from build123d import *

# Parameters (mm, degrees)
SKETCH1_R           = 48.26
SKETCH1_R_2         = 41.275
BOSS_EXTRUDE1_DEPTH = 12.7
SKETCH2_W           = 12.7
SKETCH2_H           = 12.7
BOSS_EXTRUDE2_DEPTH = 12.7
SKETCH4_W           = 2.54
SKETCH4_H           = 44.098902666
CUT_EXTRUDE2_DEPTH  = 79.456734484
BOSS_EXTRUDE3_REACH = 128.717
BOSS_EXTRUDE3_START = 48.26
SKETCH5_W           = 60.540412833
SKETCH5_H           = 12.7
SKETCH6_W           = 46.99
SKETCH6_H           = 50.8
BOSS_EXTRUDE4_DEPTH = 12.7
SKETCH7_R           = 3.429
SKETCH7_W           = 12.7
SKETCH7_H           = 11.43
CUT_EXTRUDE3_DEPTH  = 123.012315484


with BuildPart() as part:
    # Sketch1 → Boss-Extrude1 (new body)
    with BuildSketch(Plane(origin=(0, 0, 0), x_dir=(1, 0, 0), z_dir=(0, 1, 0))):
        with Locations(Location((0, 0, 0), (0, 0, 270))):
            Circle(SKETCH1_R)
        with Locations(Location((0, 0, 0), (0, 0, 270))):
            Circle(SKETCH1_R_2, mode=Mode.SUBTRACT)
    extrude(amount=BOSS_EXTRUDE1_DEPTH)

    # Sketch2 → Boss-Extrude2 (add)
    with BuildSketch(Plane(origin=(0, 0, 0), x_dir=(1, 0, 0), z_dir=(0, 1, 0))):
        with Locations((0, 54.190412833)):
            Rectangle(SKETCH2_W, SKETCH2_H)
    extrude(amount=BOSS_EXTRUDE2_DEPTH)

    # Sketch4 → Cut-Extrude2 (cut, through all)
    with BuildSketch(Plane(origin=(0, 0, 0), x_dir=(1, 0, 0), z_dir=(0, 1, 0))):
        with Locations((0, 60.121342859)):
            Rectangle(SKETCH4_W, SKETCH4_H)
    extrude(amount=CUT_EXTRUDE2_DEPTH, mode=Mode.SUBTRACT)

    # Sketch5 → Boss-Extrude3 (add, up to next)
    with BuildSketch(Plane(origin=(0, 0, 0), x_dir=(0, 0, -1), z_dir=(1, 0, 0)).offset(BOSS_EXTRUDE3_START), mode=Mode.PRIVATE) as boss_extrude3_sk1:
        with Locations((30.270206417, 6.35)):
            Rectangle(SKETCH5_W, SKETCH5_H)
    boss_extrude3_tool1 = extrude(boss_extrude3_sk1.sketch, amount=-BOSS_EXTRUDE3_REACH, mode=Mode.PRIVATE) - part.part
    add(boss_extrude3_tool1.solids().sort_by_distance((48.26, 6.35, -30.270206))[0])

    # Sketch6 → Boss-Extrude4 (add)
    with BuildSketch(Plane(origin=(0, 12.7, 0), x_dir=(1, 0, 0), z_dir=(0, 1, 0))):
        with Locations((24.765, 85.940412833)):
            Rectangle(SKETCH6_W, SKETCH6_H)
    extrude(amount=-BOSS_EXTRUDE4_DEPTH)

    # Sketch7 → Cut-Extrude3 (cut, through all)
    with BuildSketch(Plane(origin=(0, 0, 0), x_dir=(1, 0, 0), z_dir=(0, 1, 0))):
        with Locations(Location((7.62, 104.990412833, 0), (0, 0, 270))):
            Circle(SKETCH7_R)
        with Locations(Location((20.32, 104.990412833, 0), (0, 0, 270))):
            Circle(SKETCH7_R)
        with Locations(Location((20.32, 92.290412833, 0), (0, 0, 270))):
            Circle(SKETCH7_R)
        with Locations(Location((7.62, 92.290412833, 0), (0, 0, 270))):
            Circle(SKETCH7_R)
        with Locations(Location((7.62, 79.590412833, 0), (0, 0, 270))):
            Circle(SKETCH7_R)
        with Locations(Location((20.32, 79.590412833, 0), (0, 0, 270))):
            Circle(SKETCH7_R)
        with Locations(Location((7.62, 66.890412833, 0), (0, 0, 270))):
            Circle(SKETCH7_R)
        with Locations(Location((20.32, 66.890412833, 0), (0, 0, 270))):
            Circle(SKETCH7_R)
        with Locations(Location((33.02, 104.990412833, 0), (0, 0, 270))):
            Circle(SKETCH7_R)
        with Locations(Location((33.02, 92.290412833, 0), (0, 0, 270))):
            Circle(SKETCH7_R)
        with Locations(Location((33.02, 79.590412833, 0), (0, 0, 270))):
            Circle(SKETCH7_R)
        with Locations(Location((33.02, 66.890412833, 0), (0, 0, 270))):
            Circle(SKETCH7_R)
        with Locations((20.32, 53.555412833)):
            Rectangle(SKETCH7_W, SKETCH7_H)
    extrude(amount=CUT_EXTRUDE3_DEPTH, mode=Mode.SUBTRACT)


solid = part.part
Work out the finished part from the listing and answer in its coordinate system (mm). A direction names the side the tool comes from. Give positions to 0.01 mm unless a question says otherwise; leave off trailing zeros. Order: outer loops, then holes, each group sorted by start corner. A loop starts at its lowest first (then second) coordinate and runs counter-clockwise, first axis right, second up. Notation, with made-up numbers: (39.25, 3) - (86.25, 3) arc R14 ccw to (86.25, 25) - close; hole circle Ø9 at (88.25, 52.25). An arc over 180 degrees is marked (long way). Answer as CSV lines item,"result". Start each with the question number.
Q1. The part is cut by section A-A (z = 38). Write down the section's boundary in (x, y).
Q2. Find the intervals of material crossed by L1, parallel to X at y = 7.5, z = -49; L2, parallel to X at y = 5.5, z = -102.5; L3, parallel to Z at x = 33.02, y = 6 (3 decimals), in increasing order. Write a range as [from, to].
Q3. The part is cut by section D-D (x = -30.5). Write down the section's boundary in (y, z), then the cut area to 3 significant figures.
Q4. Given pin 1 Ø4 at (x, z) = (7.62, -79.59) entering from -Y; pin 2 Ø2 at (y, z) = (2.5, -42) entering from -X; pin 3 Ø4 at (x, y) = (23.5, 3.5) entering from +Z; pin 4 Ø2 at (x, y) = (-35, 8) entering from -Z, each flat-ended and moving along its own axis, determine where each tip first touches the part or whether it passes through.
Q5. For faces 1 (the face through (1.27, 6, -76)), 2 (the face through (48.26, 6, -55)), 3 (the face through (-6.35, 6, -54)), 4 (the face through (13.97, 6, -53)), 5 (the face through (14, 0, -44)), determine the directions among +Z, -Z, +X, -X, +Y, -Y from which every point of the face is accessible in a straight line to the end or side of a thin tool.
Q6. The mould has two halves that part along Z. Classify faces 6 (the face through (26.67, 6, -53)), 7 (the face through (-1.27, 6, -51)), 8 (the face through (-4, 6, -60.54)): +Z half, -Z half, draft (parallel to the pull), parting line (faces both ways), or undercut.
Q7. The part is cut by section C-C (y = 2). Give the number of separate pieces and of enclosed holes in the cut face, then the cut area to 3 significant figures.
Q8. The part is cut by section B-B (x = 20.32). Write down the section's boundary in (y, z), then the cut area to 3 significant figures.
Check result:
1,outline,"(-29.75, 0) - (-16.11, 0) - (-16.11, 12.7) - (-29.75, 12.7) - close; (16.11, 0) - (29.75, 0) - (29.75, 12.7) - (16.11, 12.7) - close"
2,L1,"x = [-6.35, -1.27], [1.27, 13.97], [26.67, 48.26]"
2,L2,"x = [1.27, 5.26], [9.98, 17.96], [22.68, 30.66], [35.38, 48.26]"
2,L3,"z = [-111.34, -108.419], [-101.561, -95.719], [-88.861, -83.019], [-76.161, -70.319], [-63.461, -24.765], [24.765, 35.195]"
3,outline,"(0, -37.4) - (12.7, -37.4) - (12.7, -27.81) - (0, -27.81) - close; (0, 27.81) - (12.7, 27.81) - (12.7, 37.4) - (0, 37.4) - close"
3,area,"244 mm²"
4,pin 1,"passes through"
4,pin 2,"stops at x = -25.46"
4,pin 3,"stops at z = 43.21"
4,pin 4,"stops at z = -34.25"
5,face 1,"-Z, +Y, -Y"
5,face 2,"+Z, -Z, +X, +Y, -Y"
5,face 3,"-Z, -X, +Y, -Y"
5,face 4,"+Y, -Y"
5,face 5,"+Z, -Z, +X, -X, -Y"
6,face 6,"undercut"
6,face 7,"draft"
6,face 8,"-Z half"
7,separate pieces,"1"
7,enclosed holes,"13"
7,area,"4,890 mm²"
8,outline,"(0, -111.34) - (12.7, -111.34) - (12.7, -108.42) - (0, -108.42) - close; (0, -101.56) - (12.7, -101.56) - (12.7, -95.72) - (0, -95.72) - close; (0, -88.86) - (12.7, -88.86) - (12.7, -83.02) - (0, -83.02) - close; (0, -76.16) - (12.7, -76.16) - (12.7, -70.32) - (0, -70.32) - close; (0, -63.46) - (12.7, -63.46) - (12.7, -59.27) - (0, -59.27) - close; (0, -47.84) - (12.7, -47.84) - (12.7, -35.93) - (0, -35.93) - close; (0, 35.93) - (12.7, 35.93) - (12.7, 43.77) - (0, 43.77) - close"
8,area,"564 mm²"
